from build123d import *

# Parameters (mm, degrees)
FILLET1_R = 2.54


with BuildPart() as part:
    # Sketch1 → Revolve1 (revolve)
    with BuildSketch(Plane(origin=(0, 0, 0), x_dir=(0, 0, -1), z_dir=(1, 0, 0)), mode=Mode.PRIVATE) as revolve1_sk:
        Polygon((0, 14.76375), (7.9375, 14.76375), (12.7, 31.75), (20.32, 34.925), (29.21, 34.29), (29.21, 31.75), (298.45, 31.75), (303.2125, 14.76375), (311.15, 14.76375), (311.15, 3.175), (307.975, 3.175), (307.975, 11.58875), (300.805254923, 11.58875), (296.042754923, 28.575), (26.035, 28.575), (26.035, 31.333696529), (20.845500206, 31.704375086), (15.341669029, 29.411112095), (10.344745077, 11.58875), (3.175, 11.58875), (3.175, 3.175), (0, 3.175), align=None)
    revolve(revolve1_sk.sketch.rotate(Axis((0, 0, 0), (0, 0, -1)), 90), axis=Axis((0, 0, 0), (0, 0, -1)))

    # Fillet1
    fillet1_edges = [part.edges().sort_by_distance(p)[0] for p in [
        (-31.75, 0, -298.45),
        (-31.75, 0, -12.7),
    ]]
    fillet(fillet1_edges, radius=FILLET1_R)


solid = part.part
Input: part model. Units: mm. Frame: model coordinates. A direction names the side the tool comes from. Round coordinates to 2 decimals unless told otherwise and drop trailing zeros. Loops run counter-clockwise (first coordinate to the right, second up) from the corner with the lowest first, then second, coordinate; pieces in that order, holes last. Notation, with made-up numbers: (16.25, -22.75) -> (70.25, -22.75) arc R14 ccw to (70.25, -3.75) -> close; hole circle Ø3 at (6, 33). An arc over 180 degrees is marked (long way). Answer as a JSON object with one key per item and string values. Group by question number.
1) Pin query (flat end, axial travel): pin 1 (1.5 mm diameter, centred on x = -6.5, y = 16, fed in from -Z); pin 2 (1.5 mm diameter, centred on x = 23.5, y = 7.5, fed in from -Z); pin 3 (1.5 mm diameter, centred on x = 19.5, y = -18, fed in from +Z); pin 4 (5.5 mm diameter, centred on x = 0, y = 0, fed in from -Z). Return the tip coordinate at first contact, or that it passes through.
2) Section query A-A on z = -265.5. Output: boundary loops of the cut face in (x, y) (3 decimals), plus the area to 3 significant figures.
3) Draft query along Y for faces 1 (the flat face through (-2.4, 2.4, -307.975)), 2 (the conical face through (32.87, -10.35, -26.8)), 3 (the conical face through (13.6, 26.2, -15.6)), 4 (the flat face through (30.3, 10, -29.21)). Return one class per face: +Y half, -Y half, draft (parallel to the pull), parting line (faces both ways), or undercut.
4) Reachability of faces 5 (the cylindrical face through (-3.2, 14.413, -307.237)), 6 (the cylindrical face through (-28.547, -1.256, -159.149)), 7 (the cylindrical face through (-3.2, 14.413, -4.024)) from +Z, -Z, +X, -X, +Y, -Y: full face, straight path, thin tool, end or side. Return the list, or none.
5) Ray query, L1, parallel to Y at x = 0, z = -1 (3 decimals); L2, parallel to Y at x = 0, z = -87 (3 decimals); L3, parallel to Z at x = 4, y = 9 (3 decimals). Return the intervals inside material, ascending.
Reply:
{
 "1": {"pin 1": "stops at z = -302.72", "pin 2": "stops at z = -300.65", "pin 3": "stops at z = -11.03", "pin 4": "passes through"},
 "2": {"outline": "circle Ø63.5 at (0, 0); hole circle Ø57.15 at (0, 0)", "area": "602 mm2"},
 "3": {"face 1": "undercut", "face 2": "parting line", "face 3": "undercut", "face 4": "draft"},
 "4": {"face 5": "-Z", "face 6": "none", "face 7": "+Z"},
 "5": {"L1": "y = -14.764 to -3.175, 3.175 to 14.764", "L2": "y = -31.75 to -28.575, 28.575 to 31.75", "L3": "z = -311.15 to -307.975, -3.175 to 0"}
}
